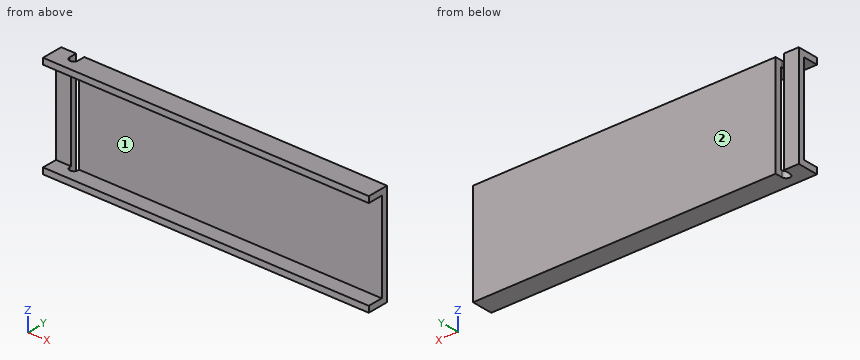
from build123d import *

# Parameters (mm, degrees)
SKETCH_1_W          = 25
SKETCH_1_H          = 10.9
SKETCH_1_W_2        = 22
SKETCH_1_H_2        = 7.9
EXTRUDE_1_DEPTH     = 80
SKETCH_3_W          = 141.586461115
SKETCH_3_H          = 11.077241851
CUT_EXTRUDE_1_DEPTH = 50


with BuildPart() as part:
    # 草图1 → 凸台-拉伸1 (new body)
    with BuildSketch(Plane(origin=(0, 0, 0), x_dir=(0, 0, -1), z_dir=(1, 0, 0))):
        with Locations((1.108975332, -0.23755131)):
            Rectangle(SKETCH_1_W, SKETCH_1_H)
        with Locations((1.108975332, -0.23755131)):
            Rectangle(SKETCH_1_W_2, SKETCH_1_H_2, mode=Mode.SUBTRACT)
    extrude(amount=EXTRUDE_1_DEPTH)

    # 草图3 → 切除-拉伸1 (cut)
    with BuildSketch(Plane.XY.offset(11.391024668)):
        with BuildLine():
            Line((3.664305979, 3.387279606), (3.664305979, 5.21244869))
            Line((3.664305979, 5.21244869), (5.664305979, 5.21244869))
            Line((5.664305979, 5.21244869), (5.664305979, 3.387279606))
            ThreePointArc((5.664305979, 3.387279606), (4.664305979, 2.387279606), (3.664305979, 3.387279606))
        make_face()
        with Locations((67.57974516, -5.538620926)):
            Rectangle(SKETCH_3_W, SKETCH_3_H)
    extrude(amount=-CUT_EXTRUDE_1_DEPTH, mode=Mode.SUBTRACT)


solid = part.part
Geometry check sheet. Reference: the model listing, model coordinates, mm. Face numbers are marked on the shaded views. A direction names the side the tool comes from. Round coordinates to 2 decimals unless told otherwise and drop trailing zeros. Loops run counter-clockwise (first coordinate to the right, second up) from the corner with the lowest first, then second, coordinate; pieces in that order, holes last.
Item 1: Cross-section at B-B on y = 1.1. Record the boundary of the cut face in (x, z).
Item 2: Cross-section at C-C on x = 60.5. Record the boundary of the cut face in (y, z).
Item 3: Thickness scan on line 1 (Z direction, x = 60.5, y = 1.25); line 2 (X direction, y = 4.6, z = -7.5); line 3 (Y direction, x = 61, z = 9.75). Record the ranges inside material, lowest first.
Item 4: Access from +Z, -Z, +X, -X, +Y, -Y to the whole of each face (thin tool, end or side, straight path). Record for the marked faces 1 and 2.
Item 5: Gauge pin test, flat end, axial feed: pin 1 (6.5 mm diameter, centred on x = 53.5, z = -2.5, fed in from -Y). Record the tip position at first contact, or that the pin passes through.
Item 6: Cross-section at A-A on z = -5.25. Record the boundary of the cut face in (x, y), then the cut area to 3 significant figures.
Answer sheet:
1. outline: (0, -13.61) - (80, -13.61) - (80, -12.11) - (0, -12.11) - close; (0, 9.89) - (80, 9.89) - (80, 11.39) - (0, 11.39) - close
2. outline: (0, -13.61) - (5.21, -13.61) - (5.21, 11.39) - (0, 11.39) - (0, 9.89) - (3.71, 9.89) - (3.71, -12.11) - (0, -12.11) - close
3. line 1: z = -13.61 to -12.11, 9.89 to 11.39
3. line 2: x = 0 to 3.66, 5.66 to 80
3. line 3: y = 3.71 to 5.21
4. face 1: +X, -X, -Y
4. face 2: +Z, -Z, +X, -X, +Y
5. pin 1: stops at y = 3.71
6. outline: (0, 3.71) - (3.66, 3.71) - (3.66, 5.21) - (0, 5.21) - close; (5.66, 3.71) - (80, 3.71) - (80, 5.21) - (5.66, 5.21) - close
6. area: 117 mm2
